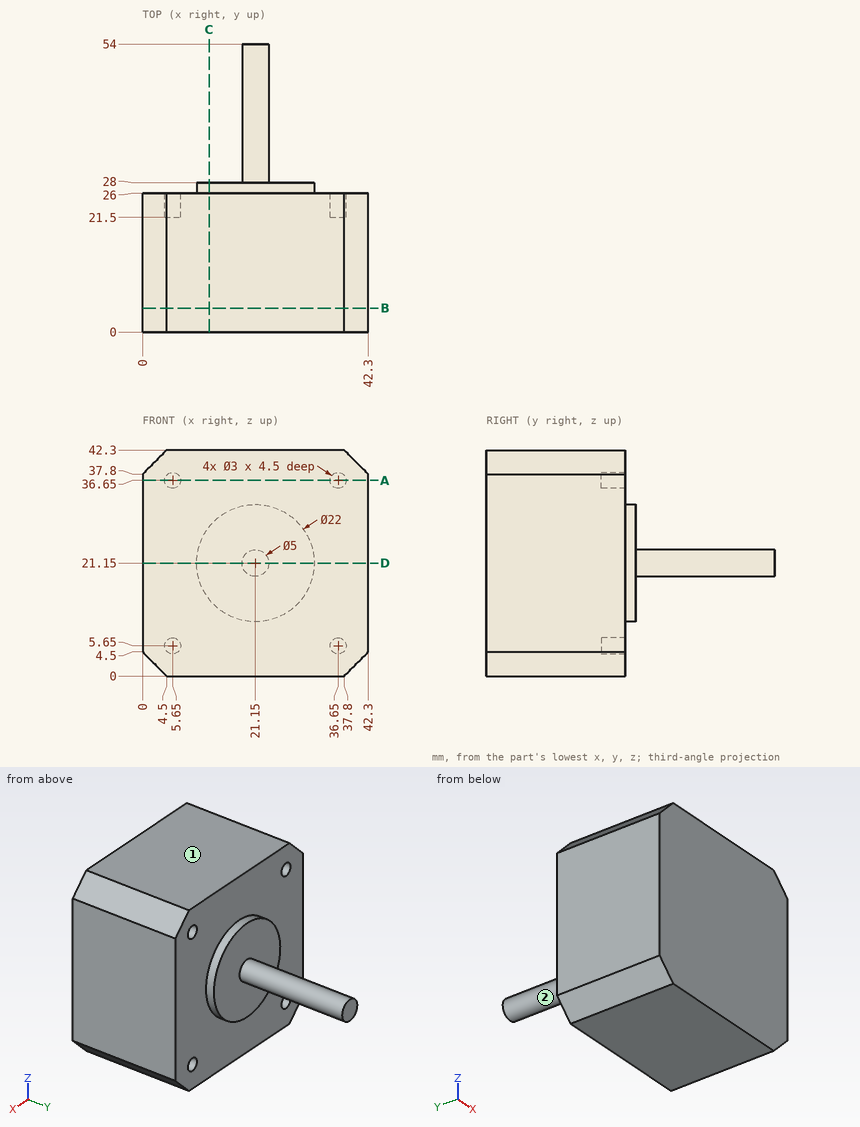
Answer from the drawing. Dimensions are ordinates in mm from the lowest x, y and z of the part. A direction names the side the tool comes from. Coordinates: 2 decimals unless noted, no trailing zeros. Write each loop counter-clockwise with the first axis right and the second up, starting at its lowest first coordinate (ties: lowest second). Pieces come first, ordered by that corner, then holes. Notation, with made-up numbers: (-0.75, 10.5) - (11.25, 10.5) arc R15 cw to (11.25, 28.5) - close; hole circle Ø4 at (77, 79). An arc over 180 degrees is marked (long way). Return JSON: item names as keys, results as strings. Group by question number.
Q1. The part is cut by section A-A on z = 36.65. Write down the section's boundary in (x, y), and give its area (3 significant figures).
Q2. Find the intervals of material crossed by line 1 along X through (y, z) = (22.7, 5.65); line 2 along Z through (x, y) = (5, 23); line 3 along Y through (x, z) = (18, 14.5), in increasing order. Write a range as [from, to].
Q3. The part is cut by section C-C on x = 12.5. Write down the section's boundary in (y, z).
Q4. The part is cut by section D-D on z = 21.15. Write down the section's boundary in (x, y).
Q5. Which of the six approach directions +Z, -Z, +X, -X, +Y, -Y give full straight-line access (tool end or side, diameter ignored) to the marked faces 1 and 2?
Q6. The part is cut by section B-B on y = 4.5. Write down the section's boundary in (x, z), and give its area (3 significant figures).
Q7. Flat-ended cylindrical pins translate along their axes: pin 1 Ø2.5 at (x, z) = (36.65, 36.65) entering from +Y; pin 2 Ø1.5 at (y, z) = (35, 19.5) entering from +X; pin 3 Ø4 at (x, z) = (5.65, 36.65) entering from +Y. Find the tip coordinate at first contact, or state that the pin passes through.
Evaluation:
{
 "1": {"outline": "(0, 0) - (42.3, 0) - (42.3, 26) - (38.15, 26) - (38.15, 21.5) - (35.15, 21.5) - (35.15, 26) - (7.15, 26) - (7.15, 21.5) - (4.15, 21.5) - (4.15, 26) - (0, 26) - close", "area": "1,070 mm2"},
 "2": {"line 1": "x = [0, 4.15], [7.15, 35.15], [38.15, 42.3]", "line 2": "z = [0, 4.3], [7, 35.3], [38, 42.3]", "line 3": "y = [0, 28]"},
 "3": {"outline": "(0, 0) - (26, 0) - (26, 14.35) - (28, 14.35) - (28, 27.95) - (26, 27.95) - (26, 42.3) - (0, 42.3) - close"},
 "4": {"outline": "(0, 0) - (42.3, 0) - (42.3, 26) - (32.15, 26) - (32.15, 28) - (23.65, 28) - (23.65, 54) - (18.65, 54) - (18.65, 28) - (10.15, 28) - (10.15, 26) - (0, 26) - close"},
 "5": {"face 1": "+Z, +X, -X, +Y, -Y", "face 2": "+Y"},
 "6": {"outline": "(0, 4.5) - (4.5, 0) - (37.8, 0) - (42.3, 4.5) - (42.3, 37.8) - (37.8, 42.3) - (4.5, 42.3) - (0, 37.8) - close", "area": "1,750 mm2"},
 "7": {"pin 1": "stops at y = 21.5", "pin 2": "stops at x = 23.48", "pin 3": "stops at y = 26"}
}
